from build123d import *

# Parameters (mm, degrees)
F0_W      = 42
F0_H      = 42
F1_DEPTH  = 4
F2_SIZE   = 7.5
F4_DEPTH  = 12
F5_SIZE   = 5
F7_DEPTH  = 13
F8_R      = 11
F9_DEPTH  = 2
F10_R     = 2.5
F11_DEPTH = 22
F12_W     = 5.2537292178
F12_H     = 0.9334036984
F13_DEPTH = 22
F14_R     = 1.5
F15_DEPTH = 6
F16_DEPTH = 25


with BuildPart() as f1:
    # F0 (on Top) → F1 (new body, symmetric)
    with BuildSketch(Plane.XY):
        Rectangle(F0_W, F0_H)
    extrude(amount=F1_DEPTH, both=True)

    # F2
    f2_edges = [f1.edges().sort_by_distance(p)[0] for p in [
        (21, 21, 0),
        (-21, 21, 0),
        (-21, -21, 0),
        (21, -21, 0),
    ]]
    chamfer(f2_edges, length=F2_SIZE)

    # F3 (on face) → F4 (join)
    with BuildSketch(Plane.XY.offset(4)):
        Polygon((13.5, 21), (-13.5, 21), (-21, 13.5), (-21, -13.5), (-13.5, -21), (13.5, -21), (21, -13.5), (21, 13.5), align=None)
        Polygon((21, 21), (13.5, 21), (21, 13.5), align=None)
        Polygon((-13.5, 21), (-21, 21), (-21, 13.5), align=None)
        Polygon((-13.5, -21), (-21, -13.5), (-21, -21), align=None)
        Polygon((21, -21), (21, -13.5), (13.5, -21), align=None)
    extrude(amount=F4_DEPTH)

    # F5
    f5_edges = [f1.edges().sort_by_distance(p)[0] for p in [
        (21, -21, 10),
        (-21, -21, 10),
        (-21, 21, 10),
        (21, 21, 10),
    ]]
    chamfer(f5_edges, length=F5_SIZE)

    # F6 (on face) → F7 (join)
    with BuildSketch(Plane(origin=(0, 0, -4), x_dir=(1, 0, 0), z_dir=(0, 0, -1))):
        Polygon((21, -16), (21, 16), (16, 21), (-16, 21), (-21, 16), (-21, -16), (-16, -21), (16, -21), align=None)
    extrude(amount=F7_DEPTH)

    # F8 (on face) → F9 (join)
    with BuildSketch(Plane.XY.offset(16)):
        Circle(F8_R)
    extrude(amount=F9_DEPTH)

    # F10 (on face) → F11 (join)
    with BuildSketch(Plane.XY.offset(18)):
        Circle(F10_R)
    extrude(amount=F11_DEPTH)

    # F12 (on face) → F13 (cut)
    with BuildSketch(Plane.XY.offset(40)):
        with Locations((-0.0065014465, 2.4667018492)):
            Rectangle(F12_W, F12_H)
    extrude(amount=-F13_DEPTH, mode=Mode.SUBTRACT)

    # F14 (on face) → F15 (cut)
    with BuildSketch(Plane.XY.offset(16)):
        with Locations((-15.5, 15.5)):
            Circle(F14_R)
        with Locations((15.5, 15.5)):
            Circle(F14_R)
        with Locations((-15.5, -15.5)):
            Circle(F14_R)
        with Locations((15.5, -15.5)):
            Circle(F14_R)
    extrude(amount=-F15_DEPTH, mode=Mode.SUBTRACT)

    # F16 (add): a face of the model
    f16_faces = [f1.faces().sort_by_distance(p)[0] for p in [
        (17.25, 17.25, 0),
    ]]
    extrude(f16_faces, amount=F16_DEPTH)


solid = f1.part
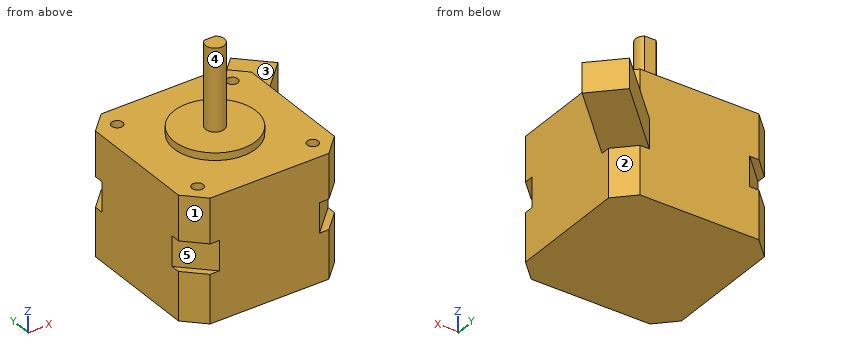
The model under review builds one solid part; all positions refer to its coordinate system, in mm. Face numbers are marked on the shaded views. A direction names the side the tool comes from. Coordinates: 2 decimals unless noted, no trailing zeros. Loops run counter-clockwise (first coordinate to the right, second up) from the corner with the lowest first, then second, coordinate; pieces in that order, holes last. Notation, with made-up numbers: M -8,-39.75 L 36,-39.75 A30 ccw 36,-4.75 Z; hole C -32.5,45 d6. An arc over 180 degrees is marked long. Put each result on its own line as item: value. Start each with the question number.
Q1. Wall thickness on line 1 (Y direction, x = 15.5, z = 14); line 2 (Y direction, x = -15, z = 14); line 3 (Z direction, x = -8, y = -2.5): over which ranges is each line inside the solid? List them lowest first.
Q2. Add section D-D (z = -13). Write out the cut boundary in (x, y), and give its area (3 significant figures).
Q3. Add section C-C (y = -6.5). Write out the cut boundary in (x, z), and give its area (3 significant figures).
Q4. Clearance check with flat-ended pins moving along their axes: pin 1 (10 mm diameter, centred on x = 12, y = 3.5, fed in from +Z); pin 2 (6 mm diameter, centred on x = -16, y = -16, fed in from +Z); pin 3 (10 mm diameter, centred on y = 20, z = -2.5, fed in from -X); pin 4 (1.5 mm diameter, centred on x = -0.5, z = 34.5, fed in from +Y). State where each tip first meets the part, or that it passes through.
Q5. Add section B-B (z = 0). Write out the cut boundary in (x, y).
Q6. For the marked faces 1, 2, 3, 4 and 5, list the 3-axis set-ups (+Z, -Z, +X, -X, +Y, -Y) from which the entire face can be reached by the end or side of a thin tool; tool diameter is ignored.
Q7. Add section A-A (x = 0). Write out the cut boundary in (y, z).
Answers:
1. line 1: y = -21 to -17, -14 to 14, 17 to 21
1. line 2: y = -21 to -16.91, -14.09 to 14.09, 16.91 to 21
1. line 3: z = -17 to 18
2. outline: M -21,-16 L -16,-21 L 16,-21 L 21,-16 L 21,16 L 16,21 L -16,21 L -21,16 Z
2. area: 1,710 mm^2
3. outline: M -21,-17 L 21,-17 L 21,16 L 8.87,16 L 8.87,18 L -8.87,18 L -8.87,16 L -21,16 Z
3. area: 1,420 mm^2
4. pin 1: stops at z = 18
4. pin 2: stops at z = 16
4. pin 3: stops at x = -21
4. pin 4: stops at y = 2
5. outline: M -21,-13.5 L -13.5,-21 L 13.5,-21 L 21,-13.5 L 21,13.5 L 38.68,31.18 L 31.18,38.68 L 13.5,21 L -13.5,21 L -21,13.5 Z
6. face 1: +Z, -Z, -X, -Y
6. face 2: -Z, +X, +Y
6. face 3: +Z, +X, +Y
6. face 4: +Z
6. face 5: -X, -Y
7. outline: M -21,-17 L 21,-17 L 21,16 L 11,16 L 11,18 L 2,18 L 2,40 L -2.5,40 L -2.5,18 L -11,18 L -11,16 L -21,16 Z
